```python
from build123d import *

# Parameters (mm, degrees)
CROQUIS1_W              = 40
CROQUIS1_H              = 25
SALIENTE_EXTRUIR2_DEPTH = 4
CORTAR_EXTRUIR1_DEPTH   = 2.8
CROQUIS3_R              = 7
SALIENTE_EXTRUIR3_DEPTH = 11
CROQUIS11_R             = 8.2
CORTAR_EXTRUIR3_DEPTH   = 9


with BuildPart() as part:
    # Croquis1 → Saliente-Extruir2 (new body)
    with BuildSketch(Plane.XY):
        with Locations((20, 12.5)):
            Rectangle(CROQUIS1_W, CROQUIS1_H)
    extrude(amount=SALIENTE_EXTRUIR2_DEPTH)

    # Croquis2 → Cortar-Extruir1 (cut)
    with BuildSketch(Plane.XY.offset(4)):
        Polygon((5, 11.881197846), (9, 14.190598923), (9, 18.809401077), (5, 21.118802154), (1, 18.809401077), (1, 14.190598923), align=None)
        Polygon((30.967302417, 14.249648614), (34.933782653, 11.883138976), (38.966480236, 14.134956805), (39.032697583, 18.753284273), (35.066217347, 21.119793911), (31.033519764, 18.867976082), align=None)
    extrude(amount=-CORTAR_EXTRUIR1_DEPTH, mode=Mode.SUBTRACT)

    # Croquis3 → Saliente-Extruir3 (add)
    with BuildSketch(Plane.XY.offset(4)):
        with BuildLine():
            Line((29.63920565, 22.043883614), (10.36079435, 22.043883614))
            ThreePointArc((10.36079435, 22.043883614), (6.694433275, 9.861459851), (14.732173124, 0))
            Line((14.732173124, 0), (25.267826876, 0))
            ThreePointArc((25.267826876, 0), (33.305566725, 9.861459851), (29.63920565, 22.043883614))
        make_face()
        with Locations((20, 12.5)):
            Circle(CROQUIS3_R, mode=Mode.SUBTRACT)
    extrude(amount=SALIENTE_EXTRUIR3_DEPTH)

    # Croquis8 → Cortar-Revolución3 (revolve, cut)
    with BuildSketch(Plane.XY.offset(10)):
        with BuildLine():
            Line((20, 25.5), (20, -0.5))
            ThreePointArc((20, -0.5), (7, 12.5), (20, 25.5))
        make_face()
    revolve(axis=Axis((20, 25.5, 10), (0, -1, 0)), mode=Mode.SUBTRACT)

    # Croquis11 → Cortar-Extruir3 (cut)
    with BuildSketch(Plane(origin=(0, 0, 0), x_dir=(-1, 0, 0), z_dir=(0, 0, -1))):
        with Locations((-20, 12.5)):
            Circle(CROQUIS11_R)
    extrude(amount=-CORTAR_EXTRUIR3_DEPTH, mode=Mode.SUBTRACT)


solid = part.part
```
Geometry check sheet. Reference: the model listing, model coordinates, mm. A direction names the side the tool comes from. Coordinates: 2 decimals unless noted, no trailing zeros. Write each loop counter-clockwise with the first axis right and the second up, starting at its lowest first coordinate (ties: lowest second). Pieces come first, ordered by that corner, then holes. Notation, with made-up numbers: M 79,-6 L 106,-6 A17 cw 106,10 Z; hole C 48.25,14.5 d5. An arc over 180 degrees is marked long. Answer as a JSON object with one key per item and string values.
1. Scan lines: L1, parallel to Y at x = 9.5, z = 13; L2, parallel to Z at x = 35.5, y = 7; L3, parallel to Y at x = 28.5, z = 6.5. Record each from-to range of solid material in increasing order.
Answers below:
{"L1": "y = 3.91 to 5.45, 19.55 to 21.09", "L2": "z = 0 to 4", "L3": "y = 1.93 to 3.31, 21.69 to 22.04"}
2. Tool access check on faces 4 (the flat face through (29, 22.044, 9)), 5 (the flat face through (5, 17, 1.2)), 6 (the flat face through (37.08, 19.92, 2.62)), 7 (the flat face through (29, 13, 0)). Record the directions out of +Z, -Z, +X, -X, +Y, -Y that give a thin tool (end or side, any length) a straight path to the whole face; none if there is none.
Answers below:
{"face 4": "+Z, +X, -X, +Y", "face 5": "none", "face 6": "+Z", "face 7": "-Z, +X, -X, +Y, -Y"}
3. Section check B-B, the plane y = 10.5. Enter the section's corners in (x, z), plus the area to 3 significant figures.
Answers below:
{"outline": "M 0,0 L 11.94,0 A12.85 cw 8.17,15 L 6.58,15 L 6.58,4 L 0,4 Z; M 28.06,0 L 40,0 L 40,4 L 33.42,4 L 33.42,15 L 31.83,15 A12.85 cw Z", "area": "102 mm²"}
4. Draft check along X on faces 1 (the cylindrical face through (33.27, 9.68, 9.42)), 2 (the flat face through (35, 17, 1.2)), 3 (the flat face through (19.7, 0, 5.7)). Enter one of: released by +X, released by -X, zero draft, split by the parting line, or undercut.
Answers below:
{"face 1": "released by +X", "face 2": "undercut", "face 3": "zero draft"}
5. Section check D-D, the plane z = 2.25. Enter the section's corners in (x, y), plus the area to 3 significant figures.
Answers below:
{"outline": "M 0,0 L 40,0 L 40,25 L 0,25 Z; hole M 1,14.19 L 5,11.88 L 9,14.19 L 9,18.81 L 5,21.12 L 1,18.81 Z; hole C 20,12.5 d20.87; hole M 30.97,14.25 L 34.93,11.88 L 38.97,14.13 L 39.03,18.75 L 35.07,21.12 L 31.03,18.87 Z", "area": "547 mm²"}
6. Section check A-A, the plane z = 11.25. Enter the section's corners in (x, y), plus the area to 3 significant figures.
Answers below:
{"outline": "M 10.36,22.04 A13.56 ccw 14.73,0 L 16.66,0 A12.94 cw 11.26,22.04 Z; M 23.34,0 L 25.27,0 A13.56 ccw 29.64,22.04 L 28.74,22.04 A12.94 cw Z", "area": "33.8 mm²"}
7. Section check C-C, the plane x = 16. Enter the section's corners in (y, z), plus the area to 3 significant figures.
Answers below:
{"outline": "M 0,0 L 5.22,0 A12.37 cw 1.19,15 L 0,15 Z; M 19.78,0 L 25,0 L 25,4 L 23.32,4 A12.37 cw Z", "area": "31.7 mm²"}
8. Go/stop test with flat-tipped pins: pin 1 Ø1.5 at (y, z) = (7, 12.5) entering from -X; pin 2 Ø1.5 at (x, z) = (31, 9.5) entering from +Y; pin 3 Ø3.5 at (x, z) = (28.5, 7) entering from +Y. Record where each tip stops, or that it passes through.
Answers below:
{"pin 1": "stops at x = 7.29", "pin 2": "stops at y = 21.38", "pin 3": "stops at y = 22.04"}
